Read the model definition and answer for the solid it produces. Units are mm, in the model's axes. Face numbers are marked on the shaded views. A direction names the side the tool comes from. Coordinates: 2 decimals unless noted, no trailing zeros. Write each loop counter-clockwise with the first axis right and the second up, starting at its lowest first coordinate (ties: lowest second). Pieces come first, ordered by that corner, then holes.
(1) Section B-B on y = 15 is taken. Write down the section's boundary in (x, z), then the cut area to 3 significant figures.
(2) Given pin 1 (1.5 mm diameter, centred on x = 3, y = -6.5, fed in from +Z); pin 2 (3 mm diameter, centred on x = -2.5, z = -5.5, fed in from +Y); pin 3 (1.7 mm diameter, centred on x = 1, y = 13.5, fed in from +Z), each flat-ended and moving along its own axis, determine where each tip first touches the part or whether it passes through.
(3) Section A-A on x = 0 is taken. Write down the section's boundary in (y, z).
(4) Section C-C on z = 0 is taken. Write down the section's boundary in (x, y).
(5) The mould has two halves that part along X. Classify the marked faces 4, 5 and 6: +X half, -X half, draft (parallel to the pull), parting line (faces both ways), or undercut.
(6) Section D-D on y = 11 is taken. Write down the section's boundary in (x, z), then the cut area to 3 significant figures.
(7) Find the intervals of material crossed by probe 1 along Y at (x, z) = (0, -0.1); probe 2 along Y at (x, z) = (5.75, -2.25); probe 3 along Y at (x, z) = (3.75, 2.5), in increasing order.
(8) Which of the six approach directions +Z, -Z, +X, -X, +Y, -Y give full straight-line access (tool end or side, diameter ignored) to the marked faces 1, 2 and 3?
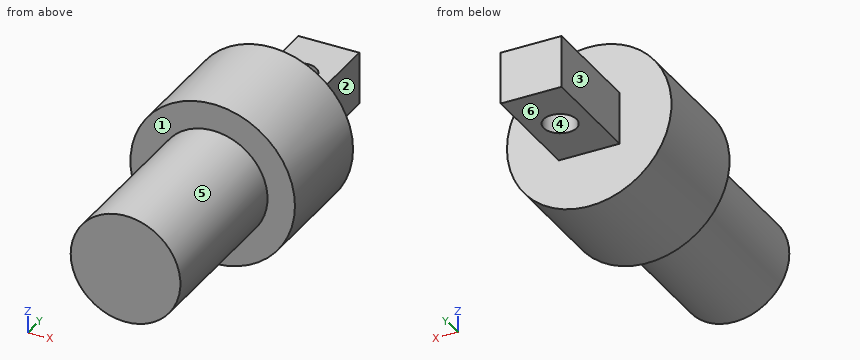
from build123d import *

# Parameters (mm, degrees)
SKETCH1_R           = 7.5
BOSS_EXTRUDE1_DEPTH = 10
SKETCH2_W           = 5.547326656
SKETCH2_H           = 4.788218798
BOSS_EXTRUDE2_DEPTH = 10
SKETCH4_R           = 1.5
CUT_EXTRUDE1_DEPTH  = 10
SKETCH5_R           = 5
BOSS_EXTRUDE3_DEPTH = 15


with BuildPart() as part:
    # Sketch1 → Boss-Extrude1 (new body)
    with BuildSketch(Plane(origin=(0, 0, 0), x_dir=(1, 0, 0), z_dir=(0, 1, 0))):
        Circle(SKETCH1_R)
    extrude(amount=BOSS_EXTRUDE1_DEPTH)

    # Sketch2 → Boss-Extrude2 (add)
    with BuildSketch(Plane(origin=(0, 10, 0), x_dir=(1, 0, 0), z_dir=(0, 1, 0))):
        Rectangle(SKETCH2_W, SKETCH2_H)
    extrude(amount=BOSS_EXTRUDE2_DEPTH)

    # Sketch4 → Cut-Extrude1 (cut)
    with BuildSketch(Plane(origin=(0, 0, -2.394109399), x_dir=(-1, 0, 0), z_dir=(0, 0, -1))):
        with Locations((0, 15)):
            Circle(SKETCH4_R)
    extrude(amount=-CUT_EXTRUDE1_DEPTH, mode=Mode.SUBTRACT)

    # Sketch5 → Boss-Extrude3 (add)
    with BuildSketch(Plane(origin=(0, 0, 0), x_dir=(-1, 0, 0), z_dir=(0, -1, 0))):
        Circle(SKETCH5_R)
    extrude(amount=BOSS_EXTRUDE3_DEPTH)


solid = part.part
Response:
1. outline: (-2.77, -2.39) - (-1.5, -2.39) - (-1.5, 2.39) - (-2.77, 2.39) - close; (1.5, -2.39) - (2.77, -2.39) - (2.77, 2.39) - (1.5, 2.39) - close
1. area: 12.2 mm2
2. pin 1: stops at z = 4.47
2. pin 2: stops at y = 10
2. pin 3: stops at z = 2.39
3. outline: (-15, -5) - (0, -5) - (0, -7.5) - (10, -7.5) - (10, -2.39) - (13.5, -2.39) - (13.5, 2.39) - (10, 2.39) - (10, 7.5) - (0, 7.5) - (0, 5) - (-15, 5) - close; (16.5, -2.39) - (20, -2.39) - (20, 2.39) - (16.5, 2.39) - close
4. outline: (-7.5, 0) - (-5, 0) - (-5, -15) - (5, -15) - (5, 0) - (7.5, 0) - (7.5, 10) - (2.77, 10) - (2.77, 20) - (-2.77, 20) - (-2.77, 10) - (-7.5, 10) - close; hole circle Ø3 at (0, 15)
5. face 4: undercut
5. face 5: parting line
5. face 6: draft
6. outline: (-2.77, -2.39) - (2.77, -2.39) - (2.77, 2.39) - (-2.77, 2.39) - close
6. area: 26.6 mm2
7. probe 1: y = -15 to 13.5, 16.5 to 20
7. probe 2: y = 0 to 10
7. probe 3: y = -15 to 10
8. face 1: -Y
8. face 2: +Z, -Z, +X, +Y
8. face 3: +Z, -Z, -X, +Y
